The figure shows three views and two pictorial views of one solid part (mm, origin at its lowest corner). Answer the questions. A direction names the side the tool comes from. Coordinates: 2 decimals unless noted, no trailing zeros. Order: outer loops, then holes, each group sorted by start corner. A loop starts at its lowest first (then second) coordinate and runs counter-clockwise, first axis right, second up. Notation, with made-up numbers: (39.5, 82) - (69.5, 82) arc R18 cw to (69.5, 94) - close; hole circle Ø3 at (9.25, 67). An arc over 180 degrees is marked (long way). Use one line per item in the form item = value.
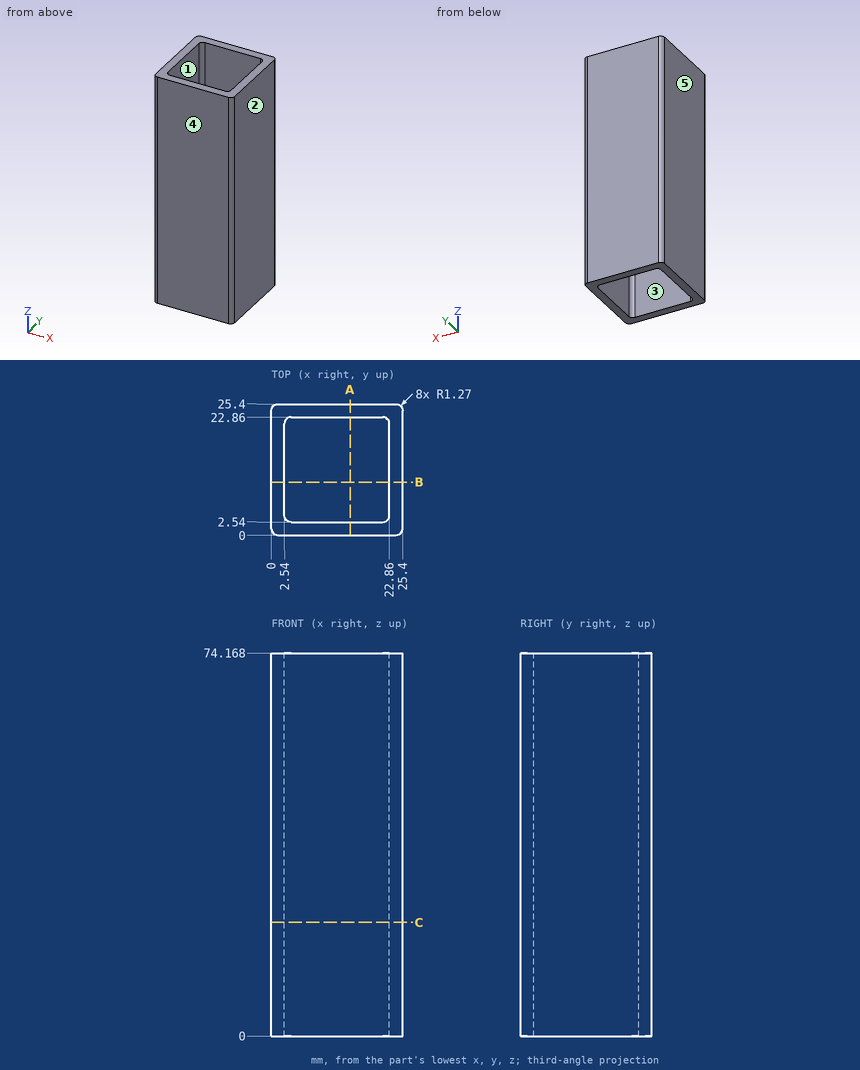
(1) Section C-C, the plane z = 22 is taken. Write down the section's boundary in (x, y).
Answer list:
outline = (0, 1.27) arc R1.27 ccw to (1.27, 0) - (24.13, 0) arc R1.27 ccw to (25.4, 1.27) - (25.4, 24.13) arc R1.27 ccw to (24.13, 25.4) - (1.27, 25.4) arc R1.27 ccw to (0, 24.13) - close; hole (2.54, 3.81) arc R1.27 ccw to (3.81, 2.54) - (21.59, 2.54) arc R1.27 ccw to (22.86, 3.81) - (22.86, 21.59) arc R1.27 ccw to (21.59, 22.86) - (3.81, 22.86) arc R1.27 ccw to (2.54, 21.59) - close
(2) Which of the six approach directions +Z, -Z, +X, -X, +Y, -Y give full straight-line access (tool end or side, diameter ignored) to the marked faces 1 and 2?
Answer list:
face_1 = +Z, -Z
face_2 = +Z, -Z, +X, +Y, -Y
(3) Straight lines are drawn through the part: L1, parallel to Y at x = 15.5, z = 7; L2, parallel to X at y = 24.5, z = 36.5. For each, find the intervals that lie inside material, in ascending order.
Answer list:
L1 = 0 to 2.54, 22.86 to 25.4
L2 = 0.06 to 25.34
(4) Section A-A, the plane x = 15.25 is taken. Write down the section's boundary in (y, z), then the cut area to 3 significant figures.
Answer list:
outline = (0, 0) - (2.54, 0) - (2.54, 74.17) - (0, 74.17) - close; (22.86, 0) - (25.4, 0) - (25.4, 74.17) - (22.86, 74.17) - close
area = 377 mm2
(5) The mould has two halves that part along X. Classify the marked faces 3, 4 and 5: +X half, -X half, draft (parallel to the pull), parting line (faces both ways), or undercut.
Answer list:
face_3 = undercut
face_4 = draft
face_5 = -X half
